Autodesk Fusion 360 part; units mm, degrees
sketch "Szkic1" plane through (0, 0, 0) normal (0, 0, 1) x (1, 0, 0)
  circle A0 centre (-15, -15) radius 2
  circle A1 centre (-15, 5) radius 2
  circle A2 centre (20, 5) radius 2
  circle A3 centre (-15, 5) radius 2
  line L0 (-35, 0) -> (-35, 15)
  line L1 (-10, -40) -> (-35, -40)
  circle A4 centre (20, -15) radius 2
  line L2 (-35, -40) -> (35, -40)
  circle A5 centre (-15, -15) radius 2
  line L3 (-35, 15) -> (-10, 15)
  line L4 (35, -40) -> (35, 15)
  line L5 (-35, -40) -> (-35, 0)
  line L6 (-35, 15) -> (-35, -40)
  line L7 (35, 15) -> (-35, 15)
  line L8 (-10, 15) -> (-10, -40)
  line L9 (-35, -40) -> (-35, -250)
  line L10 (35, -40) -> (35, -250)
  line L11 (-35, -250) -> (35, -250)
  circle A6 centre (-25, -240) radius 1.75
  circle A7 centre (25, -240) radius 1.75
  circle A8 centre (-25, -190) radius 1.75
  circle A9 centre (-25, -140) radius 1.75
  circle A10 centre (-25, -90) radius 1.75
  circle A11 centre (-25, -40) radius 1.75
  dimension "d10" = 4
  dimension "d11" = 4
  dimension "d12" = 4
  dimension "d13" = 210
  dimension "d14" = 210
  dimension "d15" = 3.5
  dimension "d16" = 3.5
  dimension "d17" = 3.5
  dimension "d18" = 3.5
  dimension "d19" = 3.5
  dimension "d20" = 3.5
extrude "Wyciągnięcie proste1" add sketch "Szkic1" along normal blind 10 contours L0 L1 L2 L3 L5 L6 L7 L8 A11 | L1 L2 L9 L10 L11 A11 | L2 L4 L7 L8
extrude "Wyciągnięcie proste2" add 1 faces at (35, -73.3333, 3.3333) along direction (1, 0, 0) blind 10
sketch "Szkic2" plane through (0, 0, 0) normal (0, 0, -1) x (1, 0, 0)
  circle A0 centre (-25, 240) radius 1.75
  circle A1 centre (-25, 190) radius 1.75
  circle A2 centre (-25, 40) radius 1.75
  circle A3 centre (25, 240) radius 1.75
  circle A4 centre (20, -5) radius 2
  circle A5 centre (-25, 90) radius 1.75
  circle A6 centre (-15, 15) radius 2
  circle A7 centre (-25, 140) radius 1.75
  circle A8 centre (-15, -5) radius 2
  circle A9 centre (20, 15) radius 2
  line L0 (45, 250) -> (-35, 250)
  line L1 (-35, 250) -> (-35, -15)
  line L2 (-35, -15) -> (45, -15)
  line L3 (45, -15) -> (45, 250)
  circle A10 centre (-15, -5) radius 3.5
  circle A11 centre (20, -5) radius 3.5
  circle A12 centre (-15, 15) radius 3.5
  circle A13 centre (20, 15) radius 3.5
  dimension "d25" = 7
  dimension "d26" = 7
  dimension "d27" = 7
  dimension "d28" = 7
extrude "Wyciągnięcie proste3" cut sketch "Szkic2" against normal blind 5 contours A10 | A11 | A12 | A13
sketch "Szkic3" plane through (0, 0, 10) normal (0, 0, 1) x (-1, 0, 0)
  circle A0 centre (25, 240) radius 1.75
  circle A1 centre (25, 190) radius 1.75
  circle A2 centre (25, 40) radius 1.75
  circle A3 centre (-25, 240) radius 1.75
  circle A4 centre (-20, -5) radius 2
  circle A5 centre (25, 90) radius 1.75
  circle A6 centre (15, 15) radius 2
  circle A7 centre (25, 140) radius 1.75
  circle A8 centre (15, -5) radius 2
  circle A9 centre (-20, 15) radius 2
  line L0 (-45, -15) -> (35, -15)
  line L1 (35, -15) -> (35, 250)
  line L2 (35, 250) -> (-45, 250)
  line L3 (-45, 250) -> (-45, -15)
  circle A10 centre (-25, 240) radius 3.5
  circle A11 centre (25, 240) radius 3.5
  circle A12 centre (25, 190) radius 3.5
  circle A13 centre (25, 140) radius 3.5
  circle A14 centre (25, 90) radius 3.5
  circle A15 centre (25, 40) radius 3.5
  dimension "d31" = 7
  dimension "d32" = 7
  dimension "d33" = 7
  dimension "d34" = 7
  dimension "d35" = 7
  dimension "d36" = 7
extrude "Wyciągnięcie proste4" cut sketch "Szkic3" against normal blind 5 contours A10 | A11 | A12 | A13 | A14 | A15
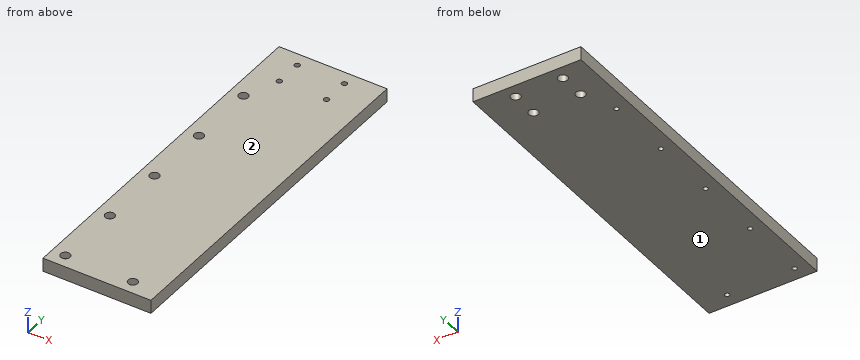
Here's how the part is built. I have some questions about the finished solid (model axes, mm). Face numbers are marked on the shaded views. Give positions to 0.01 mm unless a question says otherwise; leave off trailing zeros. Use one line per item in the form item = value. Start each with the question number.
1. If I drill on L1, parallel to X at y = -240, z = 8.55; L2, parallel to Y at x = -25, z = 1.5; L3, parallel to Y at x = -25, z = 8.35, over which ranges is the centre line in solid material (lowest first)?
2. Will these pins go through, and if not, where does the flat tip stop? pin 1 Ø3.5 at (x, y) = (-23.5, -40.5) entering from +Z; pin 2 Ø5 at (x, y) = (-15, -15) entering from -Z.
3. Thinking about a two-plate mould opening in Z: for the marked faces 1 and 2, which applies, +Z half, -Z half, draft (parallel to the pull), parting line (faces both ways), or undercut?
Entries:
q1.L1 = -35 to -28.5, -21.5 to 21.5, 28.5 to 45
q1.L2 = -250 to -241.75, -238.25 to -191.75, -188.25 to -141.75, -138.25 to -91.75, -88.25 to -41.75, -38.25 to 15
q1.L3 = -250 to -243.5, -236.5 to -193.5, -186.5 to -143.5, -136.5 to -93.5, -86.5 to -43.5, -36.5 to 15
q2.pin_1 = 5
q2.pin_2 = 5
q3.face_1 = -Z half
q3.face_2 = +Z half
